```python
from build123d import *

# Parameters (mm, degrees)
SKETCH1_R           = 5
BOSS_EXTRUDE1_DEPTH = 23
CHAMFER1_SIZE       = 0.5
CUT_EXTRUDE1_START  = -3
SKETCH2_R           = 6
SKETCH2_R_2         = 4
CUT_EXTRUDE1_DEPTH  = 1


# Read off the part's stored shape, not the designer's step: M8 Machine Threads Stud1
with BuildPart() as part:
    # Sketch1 → Boss-Extrude1 (new body)
    with BuildSketch(Plane(origin=(0, 0, 0), x_dir=(1, 0, 0), z_dir=(0, 1, 0))):
        with Locations(Location((0, 0, 0), (0, 0, 270))):
            Circle(SKETCH1_R)
    extrude(amount=BOSS_EXTRUDE1_DEPTH)

    # Chamfer1
    chamfer1_edges = [part.edges().sort_by_distance(p)[0] for p in [
        (0, 23, -5),
    ]]
    chamfer(chamfer1_edges, length=CHAMFER1_SIZE)

    # Sketch2 → Cut-Extrude1 (cut)
    with BuildSketch(Plane(origin=(0, 23, 0), x_dir=(1, 0, 0), z_dir=(0, 1, 0)).offset(CUT_EXTRUDE1_START)):
        Circle(SKETCH2_R)
        with Locations(Location((0, 0, 0), (0, 0, 270))):
            Circle(SKETCH2_R_2, mode=Mode.SUBTRACT)
    extrude(amount=-CUT_EXTRUDE1_DEPTH, mode=Mode.SUBTRACT)

    # M8 Machine Threads Stud1 outline → M8 Machine Threads Stud1 (revolve, cut)
    with BuildSketch(Plane.XY):
        Polygon((3.3095, 0), (5, 0), (5, 8), (4, 8), (4, 0.6905), align=None)
    revolve(axis=Axis((0, 0, 0), (0, 1, 0)), mode=Mode.SUBTRACT)


solid = part.part
```
Work out the finished part from the listing and answer in its coordinate system (mm). A direction names the side the tool comes from. Give positions to 0.01 mm unless a question says otherwise; leave off trailing zeros. Loops run counter-clockwise (first coordinate to the right, second up) from the corner with the lowest first, then second, coordinate; pieces in that order, holes last. Notation, with made-up numbers: (75.25, 55.25) -> (102.25, 55.25) arc R25 ccw to (102.25, 94.25) -> close; hole circle Ø10 at (25.25, 9). An arc over 180 degrees is marked (long way). Use CSV: the item, a comma, the result in double quotes.
1. A tool of negligible diameter and unlimited length cuts with its end or side. For faces 4 (the cylindrical face through (1.5, 13.42, 4.77)), 5 (the cylindrical face through (-0.867, 4.294, 3.905)), from which of +Z, -Z, +X, -X, +Y, -Y can it reach the whole face along a straight path? Write none if from no direction.
Found:
face 4,"+Y, -Y"
face 5,"-Y"
2. The part is cut by section C-C (y = 18). Write down the section's boundary in (x, z), then the cut area to 3 significant figures.
Found:
outline,"circle Ø10 at (0, 0)"
area,"78.5 mm^2"
3. The part is cut by section D-D (y = 6). Write down the section's boundary in (x, z), then the cut area to 3 significant figures.
Found:
outline,"circle Ø8 at (0, 0)"
area,"50.3 mm^2"
4. The part is cut by section A-A (x = 0). Write down the section's boundary in (y, z), then the cut area to 3 significant figures.
Found:
outline,"(0, -3.31) -> (0.69, -4) -> (8, -4) -> (8, -5) -> (19, -5) -> (19, -4) -> (20, -4) -> (20, -5) -> (22.5, -5) -> (23, -4.5) -> (23, 4.5) -> (22.5, 5) -> (20, 5) -> (20, 4) -> (19, 4) -> (19, 5) -> (8, 5) -> (8, 4) -> (0.69, 4) -> (0, 3.31) -> close"
area,"211 mm^2"
5. Flat-ended cylindrical pins translate along their axes: pin 1 Ø1 at (y, z) = (10.5, 3.5) entering from -X; pin 2 Ø2 at (y, z) = (19.5, 0) entering from -X; pin 3 Ø6 at (y, z) = (9.5, 4) entering from -X; pin 4 Ø1.5 at (x, y) = (3.5, 14.5) entering from -Z. Find the tip coordinate at first contact, or state that the pin passes through.
Found:
pin 1,"x = -4"
pin 2,"x = -5"
pin 3,"x = -4.9"
pin 4,"z = -4.18"
6. The mould has two halves that part along Y. Classify faces 1 (the flat face through (0, 0, 0)), 2 (the cylindrical face through (-4.88, 21.23, -1.08)), 3 (the cylindrical face through (-3.905, 19.507, -0.867)): +Y half, -Y half, draft (parallel to the pull), parting line (faces both ways), or undercut.
Found:
face 1,"-Y half"
face 2,"draft"
face 3,"undercut"
7. The part is cut by section B-B (z = 0). Write down the section's boundary in (x, y), then the cut area to 3 significant figures.
Found:
outline,"(-5, 8) -> (-4, 8) -> (-4, 0.69) -> (-3.31, 0) -> (3.31, 0) -> (4, 0.69) -> (4, 8) -> (5, 8) -> (5, 19) -> (4, 19) -> (4, 20) -> (5, 20) -> (5, 22.5) -> (4.5, 23) -> (-4.5, 23) -> (-5, 22.5) -> (-5, 20) -> (-4, 20) -> (-4, 19) -> (-5, 19) -> close"
area,"211 mm^2"
8. Straight lines are drawn through the part: line 1 (Y direction, x = 1.75, z = 4); line 2 (X direction, y = 18.25, z = -3); line 3 (Z direction, x = -3.75, y = 14.5). For each, find the intervals that lie inside material, in ascending order.
Found:
line 1,"8 to 19, 20 to 23"
line 2,"-4 to 4"
line 3,"-3.31 to 3.31"
